Input: part model. Units: mm. Frame: model coordinates. A direction names the side the tool comes from. Coordinates: 2 decimals unless noted, no trailing zeros. Order: outer loops, then holes, each group sorted by start corner. A loop starts at its lowest first (then second) coordinate and runs counter-clockwise, first axis right, second up.
Autodesk Inventor part; units mm, degrees
ref_plane "YZ Plane" through (0, 0, 0) normal (1, 0, 0) x (0, 1, 0)
ref_plane "XZ Plane" through (0, 0, 0) normal (0, 1, 0) x (-1, 0, 0)
ref_plane "XY Plane" through (0, 0, 0) normal (0, 0, 1) x (1, 0, 0)
sketch "Эскиз1" plane through (0, 0, 0) normal (0, 1, 0) x (-1, 0, 0)
  line L0 (-8.25, 15.4) -> (8.25, 15.4)
  line L1 (8.25, 15.4) -> (8.25, -15.4)
  line L2 (8.25, -15.4) -> (-8.25, -15.4)
  line L3 (-8.25, -15.4) -> (-8.25, 15.4)
  line L4 (-8.25, 15.4) -> (8.25, -15.4) construction
  line L5 (8.25, 15.4) -> (-8.25, -15.4) construction
  point P0 (0, 0)
  dimension "d0" = 30.8
  dimension "d1" = 16.5
extrude "Выдавливание1" add sketch "Эскиз1" along normal blind 2.5
sketch "Эскиз2" plane through (-8.25, 0, 15.4) normal (0, 0, 1) x (1, 0, 0)
  line L0 (0, 0) -> (16.5, 0) construction
  line L1 (16.5, 0) -> (16.5, 2.5) construction
  line L2 (0, 2.5) -> (16.5, 2.5) construction
  line L3 (0, 0) -> (0, 2.5) construction
  line L4 (0, 2.5) -> (0, 6)
  line L5 (0, 6) -> (1, 6)
  line L6 (0, 2.5) -> (3, 2.5)
  line L7 (0, 2.5) -> (16.5, 2.5) construction
  line L8 (3, 2.5) -> (1, 6)
  line L9 (8.25, 0) -> (8.25, 2.5) construction
  line L10 (16.5, 2.5) -> (16.5, 6)
  line L11 (16.5, 6) -> (15.5, 6)
  line L12 (16.5, 2.5) -> (13.5, 2.5)
  line L13 (13.5, 2.5) -> (15.5, 6)
  dimension "d4" = 3.5
  dimension "d5" = 1
  dimension "d6" = 3
extrude "Выдавливание2" add sketch "Эскиз2" against normal blind 25.5
sketch "Эскиз3" plane through (8.25, 0, -15.4) normal (0, 0, -1) x (-1, 0, 0)
  line L0 (0, 0) -> (16.5, 0) construction
  line L1 (16.5, 0) -> (16.5, 2.5) construction
  line L2 (0, 2.5) -> (16.5, 2.5)
  line L3 (0, 0) -> (0, 2.5) construction
  line L4 (3, 2.5) -> (0, 2.5)
  line L5 (16.5, 0) -> (16.5, 6) construction
  line L6 (0, 2.5) -> (16.5, 2.5)
  line L7 (16.5, 2.5) -> (16.5, 5)
  line L8 (16.5, 5) -> (0, 5)
  line L9 (0, 5) -> (0, 2.5)
  point P0 (8.25, 0)
  dimension "d9" = 2.5
extrude "Выдавливание3" add sketch "Эскиз3" against normal blind 3
properties part number "kicker_cover001"
Item 1: Cut plane D-D on x = 4. Return loops of the section in (y, z), then the cut area to 3 significant figures.
Response values:
outline: (0, -15.4) - (5, -15.4) - (5, -12.4) - (2.5, -12.4) - (2.5, 15.4) - (0, 15.4) - close
area: 84.5 mm2
Item 2: Draft query along X for faces 1 (the face through (-6.24, 4.23, 2.83)), 2 (the face through (0, 3, -15.4)), 3 (the face through (8.25, 3, 0)). Return one class per face: pulls with the +X half, pulls with the -X half, needs draft (parallel to the pull), parting line crosses it, or undercut.
Response values:
face 1: undercut
face 2: needs draft
face 3: pulls with the +X half
Item 3: Cut plane B-B on z = -3. Return loops of the section in (x, y).
Response values:
outline: (-8.25, 0) - (8.25, 0) - (8.25, 6) - (7.25, 6) - (5.25, 2.5) - (-5.25, 2.5) - (-7.25, 6) - (-8.25, 6) - close
Item 4: Ray query, probe 1 along Z at (x, y) = (-6, 3); probe 2 along Y at (x, z) = (2.5, -5.5); probe 3 along Z at (x, y) = (1.75, 3.25). Return the intervals inside material, ascending.
Response values:
probe 1: z = -15.4 to -12.4, -10.1 to 15.4
probe 2: y = 0 to 2.5
probe 3: z = -15.4 to -12.4
Item 5: Pin query (flat end, axial travel): pin 1 Ø0.9 at (x, z) = (3.5, -14) entering from +Y; pin 2 Ø1.2 at (x, y) = (2.5, 3.5) entering from +Z; pin 3 Ø8 at (x, z) = (1, 1) entering from +Y. Return the tip coordinate at first contact, or that it passes through.
Response values:
pin 1: stops at y = 5
pin 2: stops at z = -12.4
pin 3: stops at y = 2.5
Item 6: Cut plane C-C on x = -6.25. Return loops of the section in (y, z).
Response values:
outline: (0, -15.4) - (5, -15.4) - (5, -12.4) - (2.5, -12.4) - (2.5, -10.1) - (4.25, -10.1) - (4.25, 15.4) - (0, 15.4) - close
Item 7: Access query for faces 4 (the face through (-7, 4, -10.1)), 5 (the face through (6.24, 4.23, 2.83)), 6 (the face through (0, 5, -14)). Directions: +Z, -Z, +X, -X, +Y, -Y. A direction counts if a zero-diameter tool reaches every point of the face in a straight line with its end or side. Return the directions, or none.
Response values:
face 4: +X, -X, +Y
face 5: +Z, +Y
face 6: -Z, +X, -X, +Y
Item 8: Cut plane A-A on y = 4.5. Return loops of the section in (x, z).
Response values:
outline: (-8.25, -15.4) - (8.25, -15.4) - (8.25, -12.4) - (-8.25, -12.4) - close; (-8.25, -10.1) - (-6.39, -10.1) - (-6.39, 15.4) - (-8.25, 15.4) - close; (6.39, -10.1) - (8.25, -10.1) - (8.25, 15.4) - (6.39, 15.4) - close
